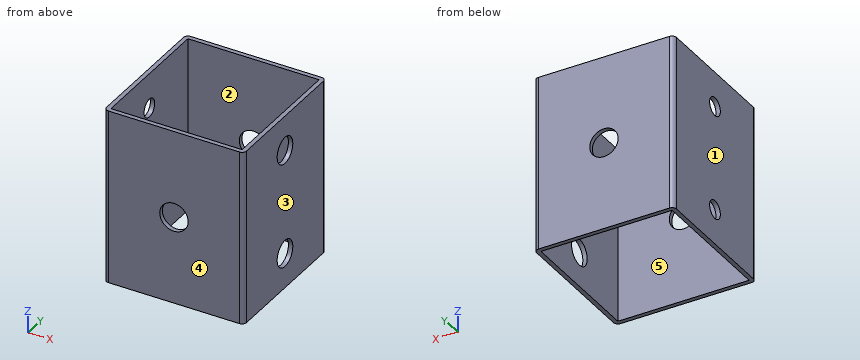
from build123d import *

# Parameters (mm, degrees)
F0_W     = 50.8
F0_H     = 50.8
F0_W_2   = 47.625
F0_H_2   = 47.625
F1_DEPTH = 63.5
F2_R     = 1.5875
F4_D     = 6.604
F6_D     = 9.652
F6_DEPTH = 12.7
F6_TIP   = 2.8997533474
F8_D     = 10.3124


with BuildPart() as f1:
    # F0 (on Top) → F1 (new body)
    with BuildSketch(Plane.XY):
        Rectangle(F0_W, F0_H)
        Rectangle(F0_W_2, F0_H_2, mode=Mode.SUBTRACT)
    extrude(amount=F1_DEPTH)

    # F2
    f2_edges = [f1.edges().sort_by_distance(p)[0] for p in [
        (25.4, -25.4, 31.75),
        (25.4, 25.4, 31.75),
        (-25.4, -25.4, 31.75),
        (-25.4, 25.4, 31.75),
    ]]
    fillet(f2_edges, radius=F2_R)

    # F4 (through all)
    with Locations(Plane.YZ.offset(25.4)):
        with Locations((0, 12.7), (0, 50.8)):
            Hole(F4_D / 2)

    # F6
    with Locations(Plane.YZ.offset(25.4)):
        with Locations((0, 50.8), (0, 12.7)):
            Hole(F6_D / 2, depth=F6_DEPTH)
            with Locations((0, 0, -(F6_DEPTH + F6_TIP / 2))):  # 118° drill point
                Cone(0, F6_D / 2, F6_TIP, mode=Mode.SUBTRACT)

    # F8 (through all)
    with Locations(Plane.XZ.offset(25.4)):
        with Locations((0, 31.75)):
            Hole(F8_D / 2)


solid = f1.part
Work out the finished part from the listing and answer in its coordinate system (mm). Face numbers are marked on the shaded views. A direction names the side the tool comes from. Round coordinates to 2 decimals unless told otherwise and drop trailing zeros. Loops run counter-clockwise (first coordinate to the right, second up) from the corner with the lowest first, then second, coordinate; pieces in that order, holes last. Notation, with made-up numbers: (63.5, 11.5) -> (121.5, 11.5) arc R28 cw to (121.5, 44.5) -> close; hole circle Ø10 at (31, -15). An arc over 180 degrees is marked (long way). Use one line per item in the form item = value.
(1) A tool of negligible diameter and unlimited length cuts with its end or side. For the marked faces 1 and 2, from which of +Z, -Z, +X, -X, +Y, -Y can it reach the whole face along a straight path? Write none if from no direction.
Answer list:
face_1 = +Z, -Z, -X, +Y, -Y
face_2 = +Z, -Z
(2) Find section B-B on z = 22. Give the vertices of the cut face in (x, y) (1 decimal), then the cut area to 3 significant figures.
Answer list:
outline = (-25.4, -23.8) arc R1.6 ccw to (-23.8, -25.4) -> (23.8, -25.4) arc R1.6 ccw to (25.4, -23.8) -> (25.4, 23.8) arc R1.6 ccw to (23.8, 25.4) -> (-23.8, 25.4) arc R1.6 ccw to (-25.4, 23.8) -> close; hole (-23.8, -23.8) -> (23.8, -23.8) -> (23.8, 23.8) -> (-23.8, 23.8) -> close
area = 310 mm2
(3) Find section A-A on y = 17. Give the vertices of the cut face in (x, z), then the cut area to 3 significant figures.
Answer list:
outline = (-25.4, 0) -> (-23.81, 0) -> (-23.81, 63.5) -> (-25.4, 63.5) -> close; (23.81, 0) -> (25.4, 0) -> (25.4, 63.5) -> (23.81, 63.5) -> close
area = 202 mm2
(4) Straight lines are drawn through the part: line 1 (Z direction, x = 24.4, y = 0); line 2 (Z direction, x = -24.5, y = 0); line 3 (Y direction, x = -0.5, z = 44.5). For each, find the intervals that lie inside material, in ascending order.
Answer list:
line_1 = 0 to 7.87, 17.53 to 45.97, 55.63 to 63.5
line_2 = 0 to 9.4, 16 to 47.5, 54.1 to 63.5
line_3 = -25.4 to -23.81, 23.81 to 25.4
(5) A flat-ended cylindrical pin translates along its axis: P1, Ø8, axis at x = 13, y = 17, coming from the -Z side. Find the tip coordinate at first contact, or state that the pin passes through.
Answer list:
P1 = through
(6) For a pull along X with two mould halves and no side action, classify the marked faces 3, 4 and 5 as released by +X, released by -X, zero draft, split by the parting line, or undercut.
Answer list:
face_3 = released by +X
face_4 = zero draft
face_5 = undercut
(7) Find section D-D on z = 50.8. Give the vertices of the cut face in (x, y) (1 decimal), then the cut area to 3 significant figures.
Answer list:
outline = (-25.4, -23.8) arc R1.6 ccw to (-23.8, -25.4) -> (23.8, -25.4) arc R1.6 ccw to (25.4, -23.8) -> (25.4, -4.8) -> (23.8, -4.8) -> (23.8, -23.8) -> (-23.8, -23.8) -> (-23.8, -3.3) -> (-25.4, -3.3) -> close; (-25.4, 3.3) -> (-23.8, 3.3) -> (-23.8, 23.8) -> (23.8, 23.8) -> (23.8, 4.8) -> (25.4, 4.8) -> (25.4, 23.8) arc R1.6 ccw to (23.8, 25.4) -> (-23.8, 25.4) arc R1.6 ccw to (-25.4, 23.8) -> close
area = 285 mm2
